Can you work these out from the model? Positions are in its coordinate system, mm. Face numbers are marked on the shaded views. A direction names the side the tool comes from. Coordinates: 2 decimals unless noted, no trailing zeros. Order: outer loops, then holes, each group sorted by start corner. A loop starts at its lowest first (then second) coordinate and runs counter-clockwise, first axis right, second up. Notation, with made-up numbers: (84, 86.25) -> (122, 86.25) arc R33 ccw to (122, 120.25) -> close; hole circle Ø5 at (-20, 22). An arc over 180 degrees is marked (long way). Answer in a Markdown table with one row per item.
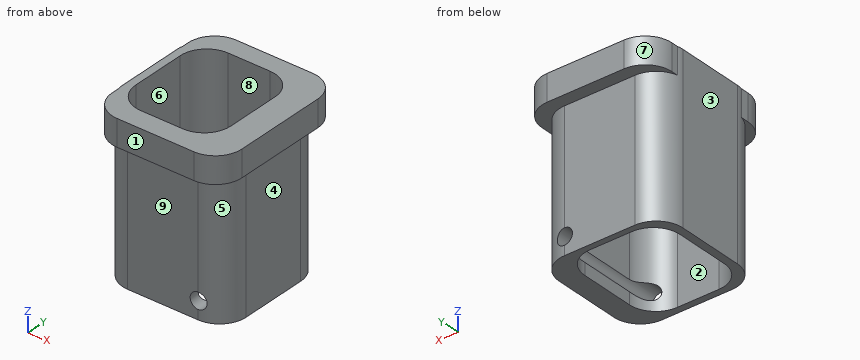
```python
from build123d import *

# Parameters (mm, degrees)
F1_DEPTH = 31
F3_DEPTH = 5
F4_DEPTH = 25
F5_R     = 1.5148959557
F6_DEPTH = 25


with BuildPart() as f1:
    # F0 (on Top) → F1 (new body)
    with BuildSketch(Plane.XY):
        with BuildLine():
            Line((7.263335404, 11.3065338519), (-6.0320308013, 11.3065338519))
            ThreePointArc((-6.0320308013, 11.3065338519), (-9.5675647072, 9.8420677578), (-11.0320308013, 6.3065338519))
            Line((-11.0320308013, 6.3065338519), (-11.0320308013, -6.3793600758))
            ThreePointArc((-11.0320308013, -6.3793600758), (-9.5675647072, -9.9148939817), (-6.0320308013, -11.3793600758))
            Line((-6.0320308013, -11.3793600758), (7.263335404, -11.3793600758))
            ThreePointArc((7.263335404, -11.3793600758), (10.7988693099, -9.9148939817), (12.263335404, -6.3793600758))
            Line((12.263335404, -6.3793600758), (12.263335404, 6.3065338519))
            ThreePointArc((12.263335404, 6.3065338519), (10.7988693099, 9.8420677578), (7.263335404, 11.3065338519))
        make_face()
        with BuildLine():
            Line((-4.572982206, 10.2046227839), (3.3416776033, 10.2046227839))
            ThreePointArc((3.3416776033, 10.2046227839), (6.8772115092, 8.7401566899), (8.3416776033, 5.2046227839))
            Line((8.3416776033, 5.2046227839), (8.3416776033, -5.13179656))
            ThreePointArc((8.3416776033, -5.13179656), (6.8772115092, -8.667330466), (3.3416776033, -10.13179656))
            Line((3.3416776033, -10.13179656), (-4.572982206, -10.13179656))
            ThreePointArc((-4.572982206, -10.13179656), (-8.1085161119, -8.667330466), (-9.572982206, -5.13179656))
            Line((-9.572982206, -5.13179656), (-9.572982206, 5.2046227839))
            ThreePointArc((-9.572982206, 5.2046227839), (-8.1085161119, 8.7401566899), (-4.572982206, 10.2046227839))
        make_face(mode=Mode.SUBTRACT)
    extrude(amount=F1_DEPTH)

    # F2 (on face) → F3 (join)
    with BuildSketch(Plane.XY.offset(31)):
        with BuildLine():
            ThreePointArc((13.5774351656, 8.6966696009), (12.1129690716, 12.2322035068), (8.5774351656, 13.6966696009))
            Line((8.5774351656, 13.6966696009), (-5.9024299309, 13.6966696009))
            ThreePointArc((-5.9024299309, 13.6966696009), (-9.4379638368, 12.2322035068), (-10.9024299309, 8.6966696009))
            Line((-10.9024299309, 8.6966696009), (-10.9024299309, -8.9936683699))
            ThreePointArc((-10.9024299309, -8.9936683699), (-9.4379638368, -12.5292022759), (-5.9024299309, -13.9936683699))
            Line((-5.9024299309, -13.9936683699), (8.5774351656, -13.9936683699))
            ThreePointArc((8.5774351656, -13.9936683699), (12.1129690716, -12.5292022759), (13.5774351656, -8.9936683699))
            Line((13.5774351656, -8.9936683699), (13.5774351656, 8.6966696009))
        make_face()
    extrude(amount=-F3_DEPTH)

    # F2 (on face) → F4 (cut)
    with BuildSketch(Plane.XY.offset(31)):
        with BuildLine():
            Line((3.3416776033, 10.2046227839), (-4.572982206, 10.2046227839))
            ThreePointArc((-4.572982206, 10.2046227839), (-8.1085161119, 8.7401566899), (-9.572982206, 5.2046227839))
            Line((-9.572982206, 5.2046227839), (-9.572982206, -5.13179656))
            ThreePointArc((-9.572982206, -5.13179656), (-8.1085161119, -8.667330466), (-4.572982206, -10.13179656))
            Line((-4.572982206, -10.13179656), (3.3416776033, -10.13179656))
            ThreePointArc((3.3416776033, -10.13179656), (6.8772115092, -8.667330466), (8.3416776033, -5.13179656))
            Line((8.3416776033, -5.13179656), (8.3416776033, 5.2046227839))
            ThreePointArc((8.3416776033, 5.2046227839), (6.8772115092, 8.7401566899), (3.3416776033, 10.2046227839))
        make_face()
    extrude(amount=-F4_DEPTH, mode=Mode.SUBTRACT)

    # F5 (on face) → F6 (cut)
    with BuildSketch(Plane.XZ.offset(11.3793600758)):
        with Locations((7.263335404, 3.3230453264)):
            Circle(F5_R)
    extrude(amount=-F6_DEPTH, mode=Mode.SUBTRACT)


solid = f1.part
```
(1) We'd pull the mould along Y, two halves only. Please class the marked faces 6, 7, 8 and 9: +Y half, -Y half, draft (parallel to the pull), parting line (faces both ways), or undercut.
Response values:
| item | result |
|---|---|
| face 6 | undercut |
| face 7 | +Y half |
| face 8 | undercut |
| face 9 | -Y half |
(2) Suppose I cut it at C-C (x = 1.75). Please give me the cut outline in (y, z).
Response values:
| item | result |
|---|---|
| outline | (-13.99, 26) -> (-11.38, 26) -> (-11.38, 0) -> (-10.13, 0) -> (-10.13, 31) -> (-13.99, 31) -> close; (10.2, 0) -> (11.31, 0) -> (11.31, 26) -> (13.7, 26) -> (13.7, 31) -> (10.2, 31) -> close |
(3) On a 3-axis mill with a long thin cutter (end or side, diameter ignored), from which of +Z, -Z, +X, -X, +Y, -Y can I reach the whole of each face in a straight line? I mean the marked faces 1, 2, 3, 4 and 5. Say none if no direction works.
Response values:
| item | result |
|---|---|
| face 1 | +Z, -Z, +X, -X, -Y |
| face 2 | +Z, -Z |
| face 3 | +Z, -Z, -X, +Y, -Y |
| face 4 | -Z, +X, +Y, -Y |
| face 5 | -Z, +X, -Y |
(4) Suppose I cut it at A-A (y = 9.75). Please give me the cut outline in (x, z).
Response values:
| item | result |
|---|---|
| outline | (-10.79, 26) -> (-9.66, 26) -> (-9.66, 0) -> (-6.66, 0) -> (-6.66, 31) -> (-10.79, 31) -> close; (5.42, 0) -> (10.89, 0) -> (10.89, 26) -> (13.47, 26) -> (13.47, 31) -> (5.42, 31) -> close; hole circle Ø3.03 at (7.26, 3.32) |
(5) Will these pins go through, and if not, where does the flat tip stop? pin 1 Ø1.2 at (y, z) = (-8.5, 28.5) entering from -X; pin 2 Ø4 at (y, z) = (0.5, 16) entering from +X; pin 3 Ø4 at (x, z) = (3, 16.5) entering from +Y.
Response values:
| item | result |
|---|---|
| pin 1 | x = -10.9 |
| pin 2 | x = 12.26 |
| pin 3 | y = 11.31 |
(6) Suppose I cut it at B-B (y = 0.5). Please give me the cut outline in (x, z), and give its area (3 significant figures).
Response values:
| item | result |
|---|---|
| outline | (-11.03, 0) -> (-9.57, 0) -> (-9.57, 31) -> (-11.03, 31) -> close; (8.34, 0) -> (12.26, 0) -> (12.26, 26) -> (13.58, 26) -> (13.58, 31) -> (8.34, 31) -> (8.34, 4.39) arc R1.51 cw to (8.34, 2.26) -> close |
| area | 173 mm2 |
(7) Suppose I cut it at D-D (z = 29.5). Please give me the cut outline in (x, y).
Response values:
| item | result |
|---|---|
| outline | (-11.03, -6.38) arc R5 ccw to (-10.9, -7.51) -> (-10.9, -8.99) arc R5 ccw to (-5.9, -13.99) -> (8.58, -13.99) arc R5 ccw to (13.58, -8.99) -> (13.58, 8.7) arc R5 ccw to (8.58, 13.7) -> (-5.9, 13.7) arc R5 ccw to (-10.9, 8.7) -> (-10.9, 7.44) arc R5 ccw to (-11.03, 6.31) -> close; hole (-9.57, -5.13) arc R5 ccw to (-4.57, -10.13) -> (3.34, -10.13) arc R5 ccw to (8.34, -5.13) -> (8.34, 5.2) arc R5 ccw to (3.34, 10.2) -> (-4.57, 10.2) arc R5 ccw to (-9.57, 5.2) -> close |
(8) I need wall thicknesses on line 1 (Y direction, x = 0.5, z = 27); line 2 (X direction, y = -3.25, z = 9.5); line 3 (Y direction, x = -1.25, z = 10). Which ranges of each line are inside material? Lowest first, please. Write a range as [from, to].
Response values:
| item | result |
|---|---|
| line 1 | [-13.99, -10.13], [10.2, 13.7] |
| line 2 | [-11.03, -9.57], [8.34, 12.26] |
| line 3 | [-11.38, -10.13], [10.2, 11.31] |
